```python
from build123d import *

# Parameters (mm, degrees)
SKETCH1_R               = 98
SKETCH1_R_2             = 78
BOSS_EXTRUDE1_DEPTH     = 20
SKETCH1_3_R             = 78
BOSS_EXTRUDE2_DEPTH     = 210
BOSS_EXTRUDE3_DEPTH     = 160
CIRPATTERN1_COUNT       = 4
BOSS_EXTRUDE4_START     = -30
SKETCH3_R               = 98
SKETCH3_R_2             = 78
BOSS_EXTRUDE4_DEPTH     = 30
SKETCH4_R               = 70
CUT_EXTRUDE1_DEPTH      = 22
SKETCH5_R               = 25
CUT_EXTRUDE2_DEPTH      = 20
CUT_EXTRUDE3_START      = -188
CUT_EXTRUDE3_OUTLINE_R  = 70
CUT_EXTRUDE3_DEPTH      = 153
SKETCH7_R               = 12.5
CUT_EXTRUDE4_DEPTH      = 218.788888605
BOSS_EXTRUDE6_DEPTH     = 90
FILLET1_R               = 10
CUT_EXTRUDE5_REACH      = 318.655
CUT_EXTRUDE5_END_RADIUS = 70
SKETCH12_R              = 5
CUT_EXTRUDE6_DEPTH      = 20


# Read off the part's stored shape, not the designer's step: Cut-Extrude3
with BuildPart() as part:
    # Sketch1 → Boss-Extrude1 (new body)
    # profile 1 of 2: a face of its own
    with BuildSketch(Plane(origin=(0, 0, 0), x_dir=(1, 0, 0), z_dir=(0, 1, 0))):
        with Locations(Location((0, 0, 0), (0, 0, 270))):
            Circle(SKETCH1_R)
        Circle(SKETCH1_R_2, mode=Mode.SUBTRACT)
    # profile 2 of 2: a face of its own
    with BuildSketch(Plane(origin=(0, 0, 0), x_dir=(1, 0, 0), z_dir=(0, 1, 0))):
        Circle(SKETCH1_R_2)
    extrude(amount=BOSS_EXTRUDE1_DEPTH)

    # Sketch1<3> → Boss-Extrude2 (add)
    with BuildSketch(Plane(origin=(0, 0, 0), x_dir=(1, 0, 0), z_dir=(0, 1, 0))):
        with Locations(Location((0, 0, 0), (0, 0, 270))):
            Circle(SKETCH1_3_R)
    extrude(amount=BOSS_EXTRUDE2_DEPTH)

    # Sketch2 → Boss-Extrude3 (add)
    with BuildSketch(Plane(origin=(0, 20, 0), x_dir=(1, 0, 0), z_dir=(0, 1, 0))):
        with BuildLine():
            ThreePointArc((9.983845423, -87.431818182), (6.867247692, -80.730824728), (-9e-09, -78))
            Line((0, -78), (0, -88))
            ThreePointArc((0, -88), (5, -87.857839718), (9.983845423, -87.431818182))
        make_face()
        with BuildLine():
            Line((0, -88), (0, -78))
            ThreePointArc((-9e-09, -78), (-6.867247699, -80.730824734), (-9.983845423, -87.431818182))
            ThreePointArc((-9.983845423, -87.431818182), (-5, -87.857839718), (0, -88))
        make_face()
        with BuildLine():
            ThreePointArc((9.983845423, -87.431818182), (5, -87.857839718), (0, -88))
            Line((0, -88), (0, -98))
            ThreePointArc((0, -98), (7.071067812, -95.071067812), (10, -88))
            ThreePointArc((10, -88), (9.99596054, -87.715794287), (9.983845423, -87.431818182))
        make_face()
        with BuildLine():
            Line((0, -98), (0, -88))
            ThreePointArc((0, -88), (-5, -87.857839718), (-9.983845423, -87.431818182))
            ThreePointArc((-9.983845423, -87.431818182), (-9.99596054, -87.715794287), (-10, -88))
            ThreePointArc((-10, -88), (-7.071067812, -95.071067812), (0, -98))
        make_face()
        with BuildLine():
            ThreePointArc((-9.983845423, -87.431818182), (-6.867247699, -80.730824734), (-9e-09, -78))
            ThreePointArc((-9e-09, -78), (-5.010347447, -77.838913266), (-10, -77.356318423))
            Line((-10, -77.356318423), (-10, -87.429971978))
            ThreePointArc((-10, -87.429971978), (-9.991922754, -87.430895453), (-9.983845423, -87.431818182))
        make_face()
        with BuildLine():
            ThreePointArc((10, -77.356318423), (5.010347438, -77.838913267), (-9e-09, -78))
            ThreePointArc((-9e-09, -78), (6.867247692, -80.730824728), (9.983845423, -87.431818182))
            ThreePointArc((9.983845423, -87.431818182), (9.991922754, -87.430895453), (10, -87.429971978))
            Line((10, -87.429971978), (10, -77.356318423))
        make_face()
    boss_extrude3 = extrude(amount=BOSS_EXTRUDE3_DEPTH)

    # CirPattern1: Boss-Extrude3 ×4 about axis
    cirpattern1_axis = Axis((0, 0, 0), (0, 1, 0))
    for i in range(1, CIRPATTERN1_COUNT):
        add(boss_extrude3.rotate(cirpattern1_axis, i * 360 / CIRPATTERN1_COUNT))

    # Sketch3 → Boss-Extrude4 (add)
    with BuildSketch(Plane(origin=(0, 210, 0), x_dir=(1, 0, 0), z_dir=(0, 1, 0)).offset(BOSS_EXTRUDE4_START)):
        with Locations(Location((0, 0, 0), (0, 0, 270))):
            Circle(SKETCH3_R)
        Circle(SKETCH3_R_2, mode=Mode.SUBTRACT)
    extrude(amount=BOSS_EXTRUDE4_DEPTH)

    # Sketch4 → Cut-Extrude1 (cut)
    with BuildSketch(Plane(origin=(0, 210, 0), x_dir=(1, 0, 0), z_dir=(0, 1, 0))):
        with Locations(Location((0, 0, 0), (0, 0, 270))):
            Circle(SKETCH4_R)
    extrude(amount=-CUT_EXTRUDE1_DEPTH, mode=Mode.SUBTRACT)

    # Sketch5 → Cut-Extrude2 (cut)
    with BuildSketch(Plane(origin=(0, 188, 0), x_dir=(1, 0, 0), z_dir=(0, 1, 0))):
        with Locations(Location((0, 0, 0), (0, 0, 270))):
            Circle(SKETCH5_R)
    extrude(amount=-CUT_EXTRUDE2_DEPTH, mode=Mode.SUBTRACT)

    # Cut-Extrude3 outline → Cut-Extrude3 (cut)
    with BuildSketch(Plane(origin=(0, 188, 0), x_dir=(1, 0, 0), z_dir=(0, 1, 0)).offset(CUT_EXTRUDE3_START)):
        Circle(CUT_EXTRUDE3_OUTLINE_R)
    extrude(amount=CUT_EXTRUDE3_DEPTH, mode=Mode.SUBTRACT)

    # Sketch7 → Cut-Extrude4 (cut, through all)
    with BuildSketch(Plane(origin=(0, 168, 0), x_dir=(1, 0, 0), z_dir=(0, 1, 0))):
        with Locations(Location((0, 0, 0), (0, 0, 270))):
            Circle(SKETCH7_R)
    extrude(amount=-CUT_EXTRUDE4_DEPTH, mode=Mode.SUBTRACT)

    # Sketch10 → Boss-Extrude6 (add)
    with BuildSketch(Plane.XZ):
        with BuildLine():
            Line((117.792189894, 0), (98, 0))
            ThreePointArc((98, 0), (93.68265963, -28.767330162), (81.111035008, -55))
            Line((81.111035008, -55), (117.792189894, -55))
            Line((117.792189894, -55), (117.792189894, 0))
        make_face()
        with BuildLine():
            ThreePointArc((81.111035008, -55), (93.68265963, -28.767330162), (98, 0))
            ThreePointArc((98, 0), (94.867247695, -7.269175269), (87.431818182, -9.983845423))
            Line((87.431818182, -9.983845423), (87.429971978, -10))
            Line((87.429971978, -10), (77.356318423, -10))
            ThreePointArc((77.356318423, -10), (70.04441747, -34.318793412), (55.308227236, -55))
            Line((55.308227236, -55), (81.111035008, -55))
        make_face()
    boss_extrude6 = extrude(amount=-BOSS_EXTRUDE6_DEPTH)

    # Mirror1: Boss-Extrude6 across plane
    add(boss_extrude6.mirror(Plane.XY))

    # Fillet1
    fillet1_edges = [part.edges().sort_by_distance(p)[0] for p in [
        (86.550208565, 90, -55),
        (86.550208565, 90, 55),
    ]]
    fillet(fillet1_edges, radius=FILLET1_R)

    # Cut-Extrude5: up to this cylinder (the profile starts outside it)
    cut_extrude5_end = Plane(origin=(0, 39.773519, 0), z_dir=(0, 1, 0)) * Cylinder(CUT_EXTRUDE5_END_RADIUS, 778.31, mode=Mode.PRIVATE)
    # Sketch11 → Cut-Extrude5 (cut, up to the surface)
    with BuildSketch(Plane(origin=(117.792189894, 0, 0), x_dir=(0, 0, -1), z_dir=(1, 0, 0)), mode=Mode.PRIVATE) as cut_extrude5_sk1:
        with BuildLine():
            Line((-45, 0), (45, 0))
            Line((45, 0), (45, 70))
            ThreePointArc((45, 70), (42.071067812, 77.071067812), (35, 80))
            Line((35, 80), (-35, 80))
            ThreePointArc((-35, 80), (-42.071067812, 77.071067812), (-45, 70))
            Line((-45, 70), (-45, 0))
        make_face()
    cut_extrude5_tool1 = extrude(cut_extrude5_sk1.sketch, amount=-CUT_EXTRUDE5_REACH, mode=Mode.PRIVATE) - cut_extrude5_end
    add(cut_extrude5_tool1.solids().sort_by_distance((117.79219, 39.773519, 0))[0], mode=Mode.SUBTRACT)

    # Sketch12 → Cut-Extrude6 (cut)
    with BuildSketch(Plane.XZ):
        with Locations(Location((-63.639610307, 63.639610307, 0), (0, 0, 270))):
            Circle(SKETCH12_R)
        with Locations(Location((63.639610307, 63.639610307, 0), (0, 0, 270))):
            Circle(SKETCH12_R)
        with Locations(Location((63.639610307, -63.639610307, 0), (0, 0, 270))):
            Circle(SKETCH12_R)
        with Locations(Location((-63.639610307, -63.639610307, 0), (0, 0, 270))):
            Circle(SKETCH12_R)
    extrude(amount=-CUT_EXTRUDE6_DEPTH, mode=Mode.SUBTRACT)


solid = part.part
```
Source: CAD feature listing. Evaluate the final solid. Frame: model axes, mm. A direction names the side the tool comes from. Round coordinates to 2 decimals unless told otherwise and drop trailing zeros. Loops run counter-clockwise (first coordinate to the right, second up) from the corner with the lowest first, then second, coordinate; pieces in that order, holes last. Notation, with made-up numbers: M -11.75,-12.5 L 33.25,-12.5 A8 ccw 33.25,-2.5 Z; hole C -6.75,81.25 d1. An arc over 180 degrees is marked long. Use a Markdown table: item, result. Add a question column.
1. Section query A-A on z = 65.5. Return the cut outline in (x, y).
2. Reachability of faces 1 (the cylindrical face through (47.12, 116.66, -62.16)), 2 (the flat face through (82, 134, 10)), 3 (the cylindrical face through (7.509, 178.14, 23.846)), 4 (the flat face through (-10, 99, -82)), 5 (the flat face through (90, 80, 0)) from +Z, -Z, +X, -X, +Y, -Y: full face, straight path, thin tool, end or side. Return the list, or none.
3. Section query C-C on y = 184. Return the cut outline in (x, z).
4. Line query: line 1 (Y direction, x = -83.5, z = 37.5); line 2 (Z direction, x = 98.5, y = 28.5); line 3 (X direction, y = 161, z = 0). Output: solid intervals per line, ascending.
5. Contact query for flat-ended pins moving along their axis: P1, Ø6, axis at x = 63.64, z = -63.64, coming from the -Y side; P2, Ø3, axis at y = 73, z = -66.5, coming from the -X side; P3, Ø4, axis at x = -31, y = 181, coming from the +Z side. Output: stop coordinate, or through.
6. Mould query, pull axis Y, two halves, no side actions, for faces 6 (the flat face through (-30, 188, -1)), 7 (the cylindrical face through (-68.52, 9.86, -62.56)), 8 (the flat face through (-82, 99, -10)). Classes: pulls with the +Y half, pulls with the -Y half, needs draft (parallel to the pull), parting line crosses it, or undercut.
7. Section query D-D on z = 39. Return the cut outline in (x, y).
8. Section query B-B on x = -36.5. Return the cut outline in (y, z), then the cut area to 3 significant figures.
Reported:
| question | item | result |
|---|---|---|
| 1 | outline | M -72.9,0 L -68.28,0 L -68.28,20 L -72.9,20 Z; M -72.9,180 L -42.35,180 L -42.35,20 L -59,20 L -59,0 L -24.69,0 L -24.69,153 L 24.69,153 L 24.69,0 L 59,0 L 59,20 L 42.35,20 L 42.35,180 L 72.9,180 L 72.9,210 L 24.69,210 L 24.69,188 L -24.69,188 L -24.69,210 L -72.9,210 Z; M 68.28,0 L 72.9,0 L 72.9,20 L 68.28,20 Z |
| 2 | face 1 | -Z, +X |
| 2 | face 2 | +Z, +X |
| 2 | face 3 | +Y |
| 2 | face 4 | -Z, -X |
| 2 | face 5 | +X, -Y |
| 3 | outline | C 0,0 d196; hole C 0,0 d50 |
| 4 | line 1 | y = 0 to 20, 180 to 210 |
| 4 | line 2 | z = -55 to -45, 45 to 55 |
| 4 | line 3 | x = -98 to -12.5, 12.5 to 98 |
| 5 | P1 | stops at y = 180 |
| 5 | P2 | stops at x = -43.12 |
| 5 | P3 | stops at z = 93.61 |
| 6 | face 6 | pulls with the +Y half |
| 6 | face 7 | needs draft |
| 6 | face 8 | undercut |
| 7 | outline | M -89.91,0 L -58.13,0 L -58.13,153 L 58.13,153 L 58.13,79.17 L 117.79,79.17 L 117.79,90 L 67.55,90 L 67.55,180 L 89.91,180 L 89.91,210 L 58.13,210 L 58.13,188 L -58.13,188 L -58.13,210 L -89.91,210 L -89.91,180 L -67.55,180 L -67.55,20 L -89.91,20 Z |
| 8 | outline | M 0,-90.95 L 20,-90.95 L 20,-68.93 L 180,-68.93 L 180,-90.95 L 210,-90.95 L 210,-59.73 L 188,-59.73 L 188,59.73 L 210,59.73 L 210,90.95 L 180,90.95 L 180,68.93 L 20,68.93 L 20,90.95 L 0,90.95 L 0,59.73 L 153,59.73 L 153,-59.73 L 0,-59.73 Z |
| 8 | area | 10,200 mm² |
